Answer from the drawing. Dimensions are ordinates in mm from the lowest x, y and z of the part. A direction names the side the tool comes from. Give positions to 0.01 mm unless a question says otherwise; leave off trailing zeros. Write each loop counter-clockwise with the first axis right and the second up, starting at its lowest first coordinate (ties: lowest second). Pieces come first, ordered by that corner, then holes.
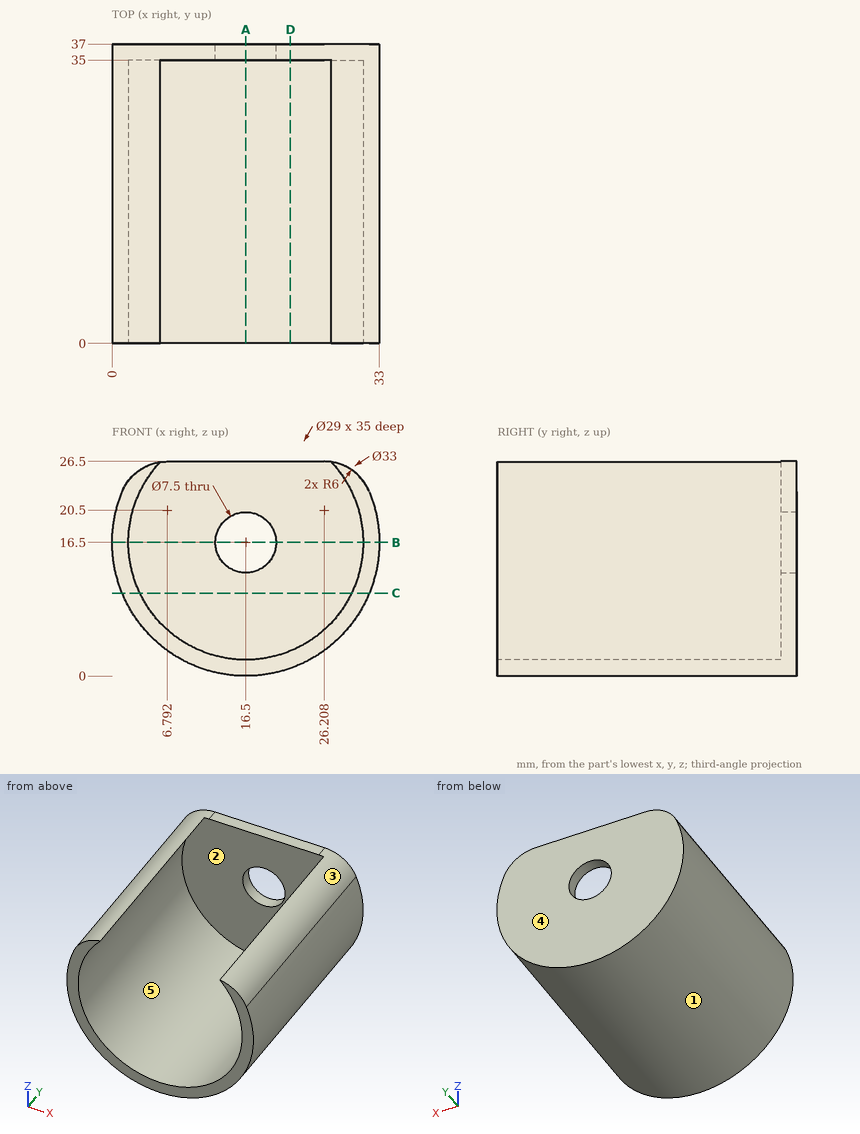
Item 1: A cutting plane is placed at C-C, the plane z = 10.25. Give the vertices of the cut face in (x, y), plus the area to 3 significant figures.
Conclusion:
outline: (1.23, 0) - (3.42, 0) - (3.42, 35) - (29.58, 35) - (29.58, 0) - (31.77, 0) - (31.77, 37) - (1.23, 37) - close
area: 214 mm2
Item 2: Which of the six approach directions +Z, -Z, +X, -X, +Y, -Y give full straight-line access (tool end or side, diameter ignored) to the marked faces 4 and 5?
Conclusion:
face 4: +Z, -Z, +X, -X, +Y
face 5: -Y
Item 3: Determine the mould class of the marked faces 1, 2 and 3 for opening direction Z: pulls with the +Z half, pulls with the -Z half, needs draft (parallel to the pull), parting line crosses it, or undercut.
Conclusion:
face 1: parting line crosses it
face 2: undercut
face 3: pulls with the +Z half
Item 4: Consider probe 1 along X at (y, z) = (26, 16.5); probe 2 along X at (y, z) = (35.6, 16.5); probe 3 along Y at (x, z) = (23.5, 18.75). Determine where each line is inside the solid, lowest interval first.
Conclusion:
probe 1: x = 0 to 2, 31 to 33
probe 2: x = 0 to 12.75, 20.25 to 33
probe 3: y = 35 to 37
Item 5: A cutting plane is placed at D-D, the plane x = 22. Give the vertices of the cut face in (y, z), plus the area to 3 significant figures.
Conclusion:
outline: (0, 0.94) - (37, 0.94) - (37, 26.5) - (35, 26.5) - (35, 3.08) - (0, 3.08) - close
area: 126 mm2
Item 6: Each of these flat-tipped pins is pushed along its axis until it touches: P1, Ø2, axis at x = 9, y = 32.5, coming from the -Z side; P2, Ø5, axis at y = 33, z = 14.5, coming from the -X side; P3, Ø2, axis at y = 24.5, z = 12.5, coming from the -X side (3 decimals); P4, Ø1, axis at y = 5.5, z = 9.5, coming from the -X side. Where does it stop, or does it pass through?
Conclusion:
P1: stops at z = 1.33
P2: stops at x = 0
P3: stops at x = 0.275
P4: stops at x = 1.33
Item 7: A cutting plane is placed at A-A, the plane x = 16.5. Give the vertices of the cut face in (y, z), plus the area to 3 significant figures.
Conclusion:
outline: (0, 0) - (37, 0) - (37, 12.75) - (35, 12.75) - (35, 2) - (0, 2) - close; (35, 20.25) - (37, 20.25) - (37, 26.5) - (35, 26.5) - close
area: 108 mm2
Item 8: A cutting plane is placed at B-B, the plane z = 16.5. Give the vertices of the cut face in (x, y), plus the area to 3 significant figures.
Conclusion:
outline: (0, 0) - (2, 0) - (2, 35) - (12.75, 35) - (12.75, 37) - (0, 37) - close; (20.25, 35) - (31, 35) - (31, 0) - (33, 0) - (33, 37) - (20.25, 37) - close
area: 191 mm2
